Autodesk Inventor part; units mm, degrees
ref_plane "YZ Plane" through (0, 0, 0) normal (1, 0, 0) x (0, 1, 0)
ref_plane "XZ Plane" through (0, 0, 0) normal (0, 1, 0) x (-1, 0, 0)
ref_plane "XY Plane" through (0, 0, 0) normal (0, 0, 1) x (1, 0, 0)
sketch "Szkic1" plane through (0, 0, 0) normal (0, 0, 1) x (1, 0, 0)
  line L0 (-40, -20.0066) -> (-24.1053, -20.0066)
  circle A0 centre (-20.0066, 0.0296) radius 3.6988
  line L1 (-24.1053, 19.9934) -> (-24.1053, 16.0243)
  line L2 (-15.8947, 19.9934) -> (-15.8947, 15.9947)
  line L3 (-40, -4.0986) -> (-35.9881, -4.0986)
  line L4 (-40, 4.1282) -> (-36.0013, 4.1282)
  line L5 (-24.1053, -20.0066) -> (-24.1053, -15.9947)
  line L6 (-15.8947, -20.0066) -> (-15.8947, -16.0079)
  line L7 (-36.0013, 10.0263) -> (-36.0013, 4.1282)
  line L8 (-35.9881, -4.0986) -> (-35.9881, -9.9967)
  line L9 (-24.1053, 16.0243) -> (-30.0033, 16.0243)
  line L10 (-24.1053, 19.9934) -> (-40, 19.9934)
  line L11 (-29.9901, -15.9947) -> (-24.1053, -15.9947)
  line L12 (-40, -20.0066) -> (-24.1053, -20.0066)
  line L13 (-27.7041, 0.0296) -> (-27.7041, 4.8995)
  line L14 (-24.8766, 7.727) -> (-20.0066, 7.727)
  line L15 (-15.0939, 7.727) -> (-20.0066, 7.727)
  line L16 (-12.2664, 4.8995) -> (-12.2664, 0.0296)
  line L17 (-12.2664, 0.0296) -> (-12.2664, -4.8832)
  line L18 (-19.9771, -7.7107) -> (-15.0939, -7.7107)
  line L19 (-19.9771, -7.7107) -> (-24.8338, -7.7107)
  line L20 (-27.7041, -4.8404) -> (-27.7041, 0.0296)
  line L21 (-30.0033, 12.8537) -> (-24.8766, 7.727)
  line L22 (-32.8308, 10.0263) -> (-27.7041, 4.8995)
  line L23 (-30.0033, 16.0243) -> (-30.0033, 12.8537)
  line L24 (-36.0013, 10.0263) -> (-32.8308, 10.0263)
  line L25 (-32.8339, -9.9967) -> (-27.7041, -4.8404)
  line L26 (-29.9901, -12.8405) -> (-24.8338, -7.7107)
  line L27 (-29.9901, -12.8405) -> (-30.0033, -12.8536)
  line L28 (-30.0033, -15.9947) -> (-29.9901, -15.9947)
  line L29 (-29.9901, -15.9947) -> (-29.9901, -12.8405)
  line L30 (-35.9881, -9.9967) -> (-32.8339, -9.9967)
  line L31 (-7.883, 9.2829) -> (-5.998, 11.1679)
  line L32 (-7.883, 9.2829) -> (-12.2664, 4.8995)
  line L33 (-10.7105, 12.1104) -> (-9.9967, 12.8242)
  line L34 (-10.7105, 12.1104) -> (-15.0939, 7.727)
  line L35 (-40, 19.9934) -> (-40, 19.9934)
  line L36 (-9.9967, 15.9947) -> (-9.9967, 12.8242)
  line L37 (0, 15.9947) -> (-1.1712, 15.9947)
  line L38 (-9.9967, 15.9947) -> (-15.8947, 15.9947)
  line L39 (-7.2141, -9.9355) -> (-5.9817, -11.1679)
  line L40 (-7.2141, -9.9355) -> (-12.2664, -4.8832)
  line L41 (-3.9823, -15.9947) -> (-5.9817, -15.9947)
  line L42 (-9.9804, -16.0079) -> (-9.9804, -12.8374)
  line L43 (-5.998, 15.9947) -> (-5.998, 11.1679)
  line L44 (-1.1712, 15.9947) -> (-5.998, 15.9947)
  line L45 (-9.9967, 15.9947) -> (-9.9804, 15.9947)
  line L46 (-5.998, -15.9947) -> (-5.9817, -15.9947)
  line L47 (-5.9817, -15.9947) -> (-5.9817, -11.1679)
  line L48 (-15.8947, -16.0079) -> (-9.9804, -16.0079)
  line L49 (-5.9817, -15.9947) -> (0, -15.9947)
  circle A1 centre (20.0066, 0.0296) radius 3.6988
  line L50 (24.1053, 19.9934) -> (24.1053, 16.0243)
  line L51 (15.9101, 19.9934) -> (15.9101, 15.9947)
  line L52 (40, -4.0986) -> (35.9881, -4.0986)
  line L53 (40, 4.1282) -> (36.0013, 4.1282)
  line L54 (24.1206, -20.0066) -> (24.1206, -15.95)
  line L55 (15.8947, -20.0066) -> (15.8947, -16.0079)
  line L56 (36.0013, 10.0263) -> (36.0013, 4.1282)
  line L57 (35.9881, -4.0986) -> (35.9881, -9.9967)
  line L58 (24.1053, 16.0243) -> (30.0186, 16.0243)
  line L59 (24.1053, 19.9934) -> (40, 19.9934)
  line L60 (30.0054, -15.95) -> (24.1206, -15.95)
  line L61 (27.7041, 0.0296) -> (27.7041, 4.8995)
  line L62 (24.8919, 7.7717) -> (20.0219, 7.7717)
  line L63 (15.1092, 7.7717) -> (20.0219, 7.7717)
  line L64 (12.2664, 4.8995) -> (12.2664, 0.0296)
  line L65 (12.2664, 0.0296) -> (12.2664, -4.8832)
  line L66 (27.7041, -4.8404) -> (27.7041, 0.0296)
  line L67 (30.0186, 12.8985) -> (24.8919, 7.7717)
  line L68 (32.8308, 10.0263) -> (27.7041, 4.8995)
  line L69 (30.0186, 16.0243) -> (30.0186, 12.8985)
  line L70 (36.0013, 10.0263) -> (32.8308, 10.0263)
  line L71 (32.8339, -9.9967) -> (27.7041, -4.8404)
  line L72 (30.0186, -15.95) -> (30.0054, -15.95)
  line L73 (35.9881, -9.9967) -> (32.8339, -9.9967)
  line L74 (7.883, 9.2829) -> (5.998, 11.1679)
  line L75 (7.883, 9.2829) -> (12.2664, 4.8995)
  line L76 (10.7258, 12.1551) -> (10.012, 12.8689)
  line L77 (10.7258, 12.1551) -> (15.1092, 7.7717)
  line L78 (40, 19.9934) -> (40, 19.9934)
  line L79 (10.012, 15.9947) -> (10.012, 12.8689)
  line L80 (0, 15.9947) -> (1.1712, 15.9947)
  line L81 (10.012, 15.9947) -> (15.9101, 15.9947)
  line L82 (7.2141, -9.9355) -> (5.9817, -11.1679)
  line L83 (7.2141, -9.9355) -> (12.2664, -4.8832)
  line L84 (10.0416, -12.7762) -> (15.0939, -7.7239)
  line L85 (3.9823, -15.9947) -> (5.9817, -15.9947)
  line L86 (9.9804, -16.0079) -> (9.9804, -12.8374)
  line L87 (10.0416, -12.7762) -> (9.9804, -12.8374)
  line L88 (5.998, 15.9947) -> (5.998, 11.1679)
  line L89 (1.1712, 15.9947) -> (5.998, 15.9947)
  line L90 (10.012, 15.9947) -> (9.9804, 15.9947)
  line L91 (5.998, -15.9947) -> (5.9817, -15.9947)
  line L92 (5.9817, -15.9947) -> (5.9817, -11.1679)
  line L93 (15.8947, -16.0079) -> (9.9804, -16.0079)
  line L94 (5.9817, -15.9947) -> (0, -15.9947)
  line L95 (0, 16.0243) -> (0, 15.9947)
  line L96 (0, -20.0066) -> (0, -19.9934)
  line L97 (0, -16.0079) -> (0, -15.9947)
  line L98 (-40, 4.1282) -> (-40, 19.9934)
  line L99 (-40, -4.0986) -> (-40, -20.0066)
  line L100 (40, 4.1282) -> (40, 19.9934)
  line L101 (40, -20.0066) -> (40, -4.0986)
  line L102 (24.1206, -20.0066) -> (40, -20.0066)
  line L103 (24.8766, -7.7239) -> (15.0939, -7.7239)
  line L104 (30.0186, -15.95) -> (30.0186, -12.8089)
  line L105 (30.0186, -12.8089) -> (24.8766, -7.7239)
  line L106 (-15.8947, -20.0066) -> (15.8947, -20.0066)
  line L107 (-9.9804, -12.8374) -> (-15.0939, -7.7107)
  line L108 (-15.8947, 19.9934) -> (15.9101, 19.9934)
  point P0 (0, 0)
  dimension "d54" = 40
  dimension "d56" = 80
  dimension "d57" = 80
  dimension "d61" = 40
  dimension "d62" = 40
  dimension "d65" = 0
  dimension "d66" = 0
extrude "Wyciągnięcie proste2" add sketch "Szkic1" along normal blind 600
properties part number "Profil aluminiowy alutec K&K 104080"
Input: part model. Units: mm. Frame: model coordinates. A direction names the side the tool comes from. Coordinates: 2 decimals unless noted, no trailing zeros. Answer as a JSON object with one key per item and string values.
1. Material intervals for line 1 (X direction, y = -14, z = 157.5); line 2 (X direction, y = 0.5, z = 521); line 3 (Y direction, x = 15, z = 527.5), sorted ascending. Write a range as from..to.
Result set:
{"line 1": "x = -40..-29.99, -9.98..-5.98, 5.98..9.98, 30.02..40", "line 2": "x = -27.7..-23.68, -16.34..-12.27, 12.27..16.34, 23.68..27.7", "line 3": "y = -20.01..-16.01, -7.82..7.88, 15.99..19.99"}
2. Mould query, pull axis Y, two halves, no side actions, for faces 1 (the face through (-32, -20.007, 296)), 2 (the face through (40, 12, 296)), 3 (the face through (-27.704, 0, 296)). Classes: released by +Y, released by -Y, zero draft, split by the parting line, or undercut.
Result set:
{"face 1": "released by -Y", "face 2": "zero draft", "face 3": "undercut"}
3. First-contact query: P1, Ø8, axis at y = 2.5, z = 186, coming from the +X side; P2, Ø5, axis at x = -20.5, z = 390, coming from the -Y side; P3, Ø1, axis at x = -19, z = 325.5, coming from the +Y side. Flat tips, straight axial feed; report the tip coordinate or a pass-through.
Result set:
{"P1": "stops at x = 40", "P2": "stops at y = -7.71", "P3": "stops at y = 7.73"}
4. Section A-A on z = 107. Count the separate pieces of the cut face and the enclosed holes in it, then the cut area to 3 significant figures.
Result set:
{"separate pieces": "1", "enclosed holes": "3", "area": "1,500 mm2"}
5. Access query for faces 4 (the face through (-9, 9, 600)), 5 (the face through (20, 7.772, 296)). Directions: +Z, -Z, +X, -X, +Y, -Y. A direction counts if a zero-diameter tool reaches every point of the face in a straight line with its end or side. Return the directions, or none.
Result set:
{"face 4": "+Z, +X, -X, +Y, -Y", "face 5": "+Z, -Z"}
